Part print with two shaded views. Sizes in mm from the minimum x, y, z corner. A direction names the side the tool comes from. Give positions to 0.01 mm unless a question says otherwise; leave off trailing zeros. Loops run counter-clockwise (first coordinate to the right, second up) from the corner with the lowest first, then second, coordinate; pieces in that order, holes last. Notation, with made-up numbers: M 3,19.5 L 51,19.5 A20 cw 51,33.5 Z; hole C -29.75,44 d6. An arc over 180 degrees is marked long. Answer as a JSON object with one key per item and string values. Group by question number.
1. 3-axis set-ups, long thin cutter, end or side, ignore diameter. For the marked faces 4, 5 and 6: which of +Z, -Z, +X, -X, +Y, -Y reach the whole face in a straight line?
2. Drill centre lines: line 1 along Y through (x, z) = (4.5, 25); line 2 along X through (y, z) = (3, 25); line 3 along Y through (x, z) = (22.5, 54). Where is each one in solid material? Low to high. Write a range as [from, to].
3. Drop flat-ended pins along their axis: pin 1 Ø4 at (x, y) = (18.5, 95) entering from -Z; pin 2 Ø8 at (x, z) = (25, 25) entering from -Y; pin 3 Ø10 at (y, z) = (22.5, 40) entering from +X; pin 4 Ø8 at (y, z) = (67.5, 54) entering from +X. Give the stop position or say it passes through.
4. Slice it at D-D (z = 6). List the corners of the cut face in (x, y), then the cut area to 3 significant figures.
5. Slice it at B-B (x = 45). List the corners of the cut face in (y, z).
6. Slice it at C-C (z = 53). List the corners of the cut face in (x, y), then the cut area to 3 significant figures.
7. Slice it at A-A (y = 22.5). List the corners of the cut face in (x, z), then the cut area to 3 significant figures.
8. Mould opens along X. For the marked faces 1, 2 and 3 say: released by +X, released by -X, zero draft, split by the parting line, or undercut.
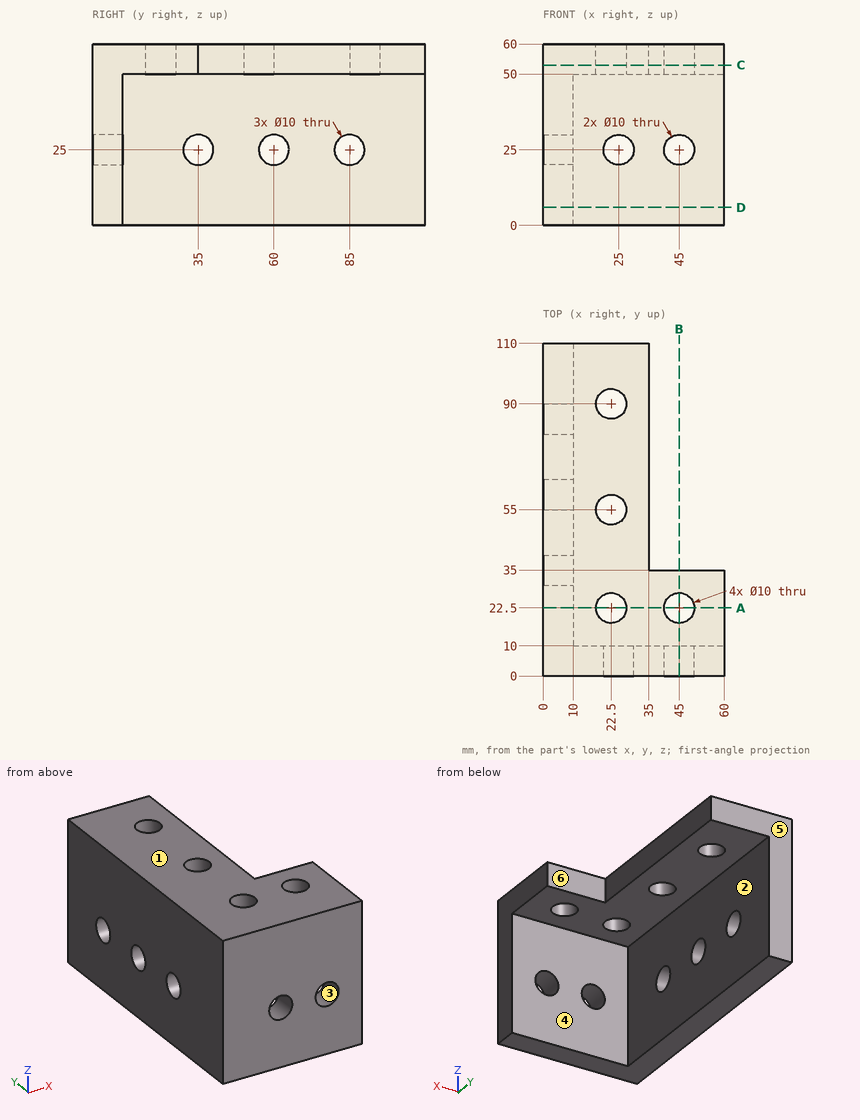
Established:
{
 "1": {"face 4": "-Z, +X, +Y", "face 5": "+Z, -Z, +X, -X, +Y", "face 6": "+Z, -Z, +X, +Y"},
 "2": {"line 1": "y = [0, 30], [40, 55], [65, 80], [90, 110]", "line 2": "x = [0, 20], [30, 40], [50, 60]", "line 3": "y = [0, 17.5], [27.5, 50], [60, 85], [95, 110]"},
 "3": {"pin 1": "stops at z = 50", "pin 2": "passes through", "pin 3": "stops at x = 10", "pin 4": "stops at x = 35"},
 "4": {"outline": "M 0,0 L 60,0 L 60,10 L 10,10 L 10,110 L 0,110 Z", "area": "1,600 mm^2"},
 "5": {"outline": "M 0,0 L 10,0 L 10,20 L 0,20 Z; M 0,30 L 10,30 L 10,50 L 17.5,50 L 17.5,60 L 0,60 Z; M 27.5,50 L 35,50 L 35,60 L 27.5,60 Z"},
 "6": {"outline": "M 0,0 L 60,0 L 60,35 L 35,35 L 35,110 L 0,110 Z; hole C 22.5,22.5 d10; hole C 22.5,55 d10; hole C 22.5,90 d10; hole C 45,22.5 d10", "area": "4,410 mm^2"},
 "7": {"outline": "M 0,0 L 10,0 L 10,50 L 17.5,50 L 17.5,60 L 0,60 Z; M 27.5,50 L 40,50 L 40,60 L 27.5,60 Z; M 50,50 L 60,50 L 60,60 L 50,60 Z", "area": "900 mm^2"},
 "8": {"face 1": "zero draft", "face 2": "released by +X", "face 3": "undercut"}
}
